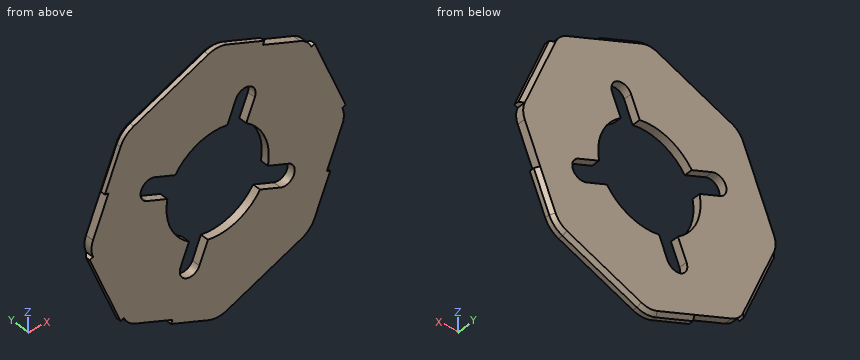
```python
from build123d import *

# Parameters (mm, degrees)
BOSS_EXTRUDE1_DEPTH = 1.6
CHAMFER1_SIZE       = 0.7
CUT_EXTRUDE1_DEPTH  = 10
CUT_EXTRUDE2_DEPTH  = 10


with BuildPart() as part:
    # Sketch1 → Boss-Extrude1 (new body)
    with BuildSketch(Plane(origin=(0, 0, 0), x_dir=(1, 0, 0), z_dir=(0, 1, 0))):
        with BuildLine():
            Line((-9.10786569, -21.988332874), (-1.836880475, -25.000073562))
            ThreePointArc((-1.836880475, -25.000073562), (0, -25.365451806), (1.836880475, -25.000073562))
            Line((1.836880475, -25.000073562), (16.378850905, -18.976592186))
            ThreePointArc((16.378850905, -18.976592186), (17.93608298, -17.93608298), (18.976592186, -16.378850905))
            Line((18.976592186, -16.378850905), (25.000073562, -1.836880475))
            ThreePointArc((25.000073562, -1.836880475), (25.365451806, 0), (25.000073562, 1.836880475))
            Line((25.000073562, 1.836880475), (18.976592186, 16.378850905))
            ThreePointArc((18.976592186, 16.378850905), (17.93608298, 17.93608298), (16.378850905, 18.976592186))
            Line((16.378850905, 18.976592186), (1.836880475, 25.000073562))
            ThreePointArc((1.836880475, 25.000073562), (0, 25.365451806), (-1.836880475, 25.000073562))
            Line((-1.836880475, 25.000073562), (-16.378850905, 18.976592186))
            ThreePointArc((-16.378850905, 18.976592186), (-17.93608298, 17.93608298), (-18.976592186, 16.378850905))
            Line((-18.976592186, 16.378850905), (-25.000073562, 1.836880475))
            ThreePointArc((-25.000073562, 1.836880475), (-25.365451806, 0), (-25.000073562, -1.836880475))
            Line((-25.000073562, -1.836880475), (-18.976592186, -16.378850905))
            ThreePointArc((-18.976592186, -16.378850905), (-17.93608298, -17.93608298), (-16.378850905, -18.976592186))
            Line((-16.378850905, -18.976592186), (-9.10786569, -21.988332874))
        make_face()
    extrude(amount=BOSS_EXTRUDE1_DEPTH)

    # Chamfer1
    chamfer1_edges = [part.edges().sort_by_distance(p)[0] for p in [
        (0, 1.6, 25.365451806),
        (9.10786569, 1.6, 21.988332874),
        (17.93608298, 1.6, 17.93608298),
        (21.988332874, 1.6, 9.10786569),
        (25.365451806, 1.6, 0),
        (21.988332874, 1.6, -9.10786569),
        (17.93608298, 1.6, -17.93608298),
        (9.10786569, 1.6, -21.988332874),
        (0, 1.6, -25.365451806),
        (-9.10786569, 1.6, -21.988332874),
        (-9.10786569, 1.6, 21.988332874),
        (-17.93608298, 1.6, -17.93608298),
        (-21.988332874, 1.6, -9.10786569),
        (-25.365451806, 1.6, 0),
        (-21.988332874, 1.6, 9.10786569),
        (-17.93608298, 1.6, 17.93608298),
    ]]
    chamfer(chamfer1_edges, length=CHAMFER1_SIZE)

    # Sketch3 → Cut-Extrude1 (cut)
    with BuildSketch(Plane(origin=(0, 1.6, 0), x_dir=(1, 0, 0), z_dir=(0, 1, 0))):
        with BuildLine():
            Line((11.184254927, -26.400355762), (8.839987288, -21.341617201))
            Line((8.839987288, -21.341617201), (16.110972503, -18.329876513))
            ThreePointArc((16.110972503, -18.329876513), (17.441108233, -17.441108233), (18.329876513, -16.110972503))
            Line((18.329876513, -16.110972503), (20.565451806, -17.036978108))
            Line((20.565451806, -17.036978108), (27.482751604, -2.865239392))
            Line((27.482751604, -2.865239392), (24.353357889, -1.569002073))
            ThreePointArc((24.353357889, -1.569002073), (24.665451806, 0), (24.353357889, 1.569002073))
            Line((24.353357889, 1.569002073), (21.341617201, 8.839987288))
            Line((21.341617201, 8.839987288), (23.946233788, 9.918854803))
            Line((23.946233788, 9.918854803), (36.794025395, -9.102301388))
            Line((36.794025395, -9.102301388), (11.184254927, -26.400355762))
        make_face()
        with BuildLine():
            Line((-8.839987288, 21.341617201), (-16.110972503, 18.329876513))
            ThreePointArc((-16.110972503, 18.329876513), (-17.441108233, 17.441108233), (-18.329876513, 16.110972503))
            Line((-18.329876513, 16.110972503), (-20.565451806, 17.036978108))
            Line((-20.565451806, 17.036978108), (-26.15363219, 2.314700104))
            Line((-26.15363219, 2.314700104), (-24.353357889, 1.569002073))
            ThreePointArc((-24.353357889, 1.569002073), (-24.665451806, 0), (-24.353357889, -1.569002073))
            Line((-24.353357889, -1.569002073), (-21.341617201, -8.839987288))
            Line((-21.341617201, -8.839987288), (-32.211044195, -10.986258031))
            Line((-32.211044195, -10.986258031), (-37.928163695, 17.967131565))
            Line((-37.928163695, 17.967131565), (-9.747163954, 23.531735412))
            Line((-9.747163954, 23.531735412), (-8.839987288, 21.341617201))
        make_face()
    extrude(amount=-CUT_EXTRUDE1_DEPTH, mode=Mode.SUBTRACT)

    # Sketch4 → Cut-Extrude2 (cut)
    with BuildSketch(Plane(origin=(0, 1.6, 0), x_dir=(1, 0, 0), z_dir=(0, 1, 0))):
        with BuildLine():
            Line((-7.259720066, 12.300262784), (-5.597275634, 8.286766889))
            ThreePointArc((-5.597275634, 8.286766889), (-9.238795325, 3.826834324), (-9.817500619, -1.901757504))
            Line((-9.817500619, -1.901757504), (-13.830996513, -3.564201936))
            ThreePointArc((-13.830996513, -3.564201936), (-14.913253575, -6.177654038), (-12.299610465, -7.259449732))
            Line((-12.299610465, -7.259449732), (-8.287642823, -5.595978595))
            ThreePointArc((-8.287642823, -5.595978595), (-3.827557299, -9.238495826), (1.901757504, -9.817500619))
            Line((1.901757504, -9.817500619), (3.564201936, -13.830996513))
            ThreePointArc((3.564201936, -13.830996513), (6.177327866, -14.913388714), (7.259720066, -12.300262784))
            Line((7.259720066, -12.300262784), (5.597275634, -8.286766889))
            ThreePointArc((5.597275634, -8.286766889), (9.240445033, -3.822849145), (9.815856456, 1.910225649))
            Line((9.815856456, 1.910225649), (14.012213043, 3.650149468))
            ThreePointArc((14.012213043, 3.650149468), (14.872687986, 6.269014189), (12.300262784, 7.259720066))
            Line((12.300262784, 7.259720066), (8.286766889, 5.597275634))
            ThreePointArc((8.286766889, 5.597275634), (3.826834324, 9.238795325), (-1.901757504, 9.817500619))
            Line((-1.901757504, 9.817500619), (-3.564201936, 13.830996513))
            ThreePointArc((-3.564201936, 13.830996513), (-6.177327866, 14.913388714), (-7.259720066, 12.300262784))
        make_face()
    extrude(amount=-CUT_EXTRUDE2_DEPTH, mode=Mode.SUBTRACT)


solid = part.part
```
Here's how the part is built. I have some questions about the finished solid (model axes, mm). Coordinates: 2 decimals unless noted, no trailing zeros. Order: outer loops, then holes, each group sorted by start corner. A loop starts at its lowest first (then second) coordinate and runs counter-clockwise, first axis right, second up.
1) Imagine slicing it at C-C on x = -6.5. List the corners of the cut face in (y, z) for me.
2) I need wall thicknesses on line 1 (Z direction, x = 6, y = 1.1); line 2 (Z direction, x = 11, y = 1.2); line 3 (X direction, y = 1.1, z = -4). Which ranges of each line are inside material? Lowest first, please.
3) Imagine slicing it at A-A on x = 11.5. List the corners of the cut face in (y, z) for me.
4) Will this pin go through, and if not, where does the flat tip stop? pin 1 (2 mm diameter, centred on x = 6.5, z = 3.5, fed in from -Y).
5) Imagine slicing it at B-B on z = -11. List the corners of the cut face in (x, y) for me.
Response values:
1. outline: (0, -23.07) - (0.9, -23.07) - (1.6, -22.31) - (1.6, -14.74) - (0, -14.74) - close; (0, -10.47) - (1.6, -10.47) - (1.6, -7.6) - (0, -7.6) - close; (0, 7.6) - (1.6, 7.6) - (1.6, 22.31) - (0.9, 23.07) - (0, 23.07) - close
2. line 1: z = -23.06 to -8, 8 to 9.26, 14.98 to 23.06
2. line 2: z = -20.88 to -6.72, -2.4 to 20.45
2. line 3: x = -23.89 to -9.17, 14.48 to 23.35
3. outline: (0, -21) - (0.9, -21) - (1.6, -20.24) - (1.6, -6.93) - (0, -6.93) - close; (0, -2.61) - (1.6, -2.61) - (1.6, 20.24) - (0, 20.24) - close
4. pin 1: passes through
5. outline: (-21.2, 0) - (-6.72, 0) - (-6.72, 1.6) - (-20.45, 1.6) - (-21.2, 0.9) - close; (-2.39, 0) - (21.2, 0) - (21.2, 0.9) - (20.45, 1.6) - (-2.39, 1.6) - close
